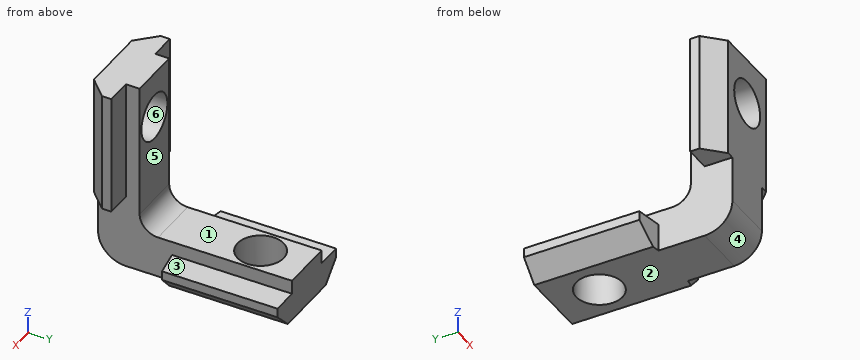
from build123d import *

# Parameters (mm, degrees)
BOSS_EXTRUDE1_DEPTH      = 13
SKETCH2_R                = 2.5
CUT_EXTRUDE1_DEPTH       = 23.207487476
BOSS_EXTRUDE2_DEPTH      = 13
CUT_EXTRUDE2_DEPTH       = 28.297847901
BOSS_EXTRUDE3_DEPTH      = 2.85
BOSS_EXTRUDE3_DEPTH_BACK = 2.85
SKETCH5_W                = 4.5
SKETCH5_H                = 2.5


with BuildPart() as part:
    # Sketch1 → Boss-Extrude1 (new body)
    with BuildSketch(Plane.XY.offset(21)):
        Polygon((-2.85, 4.5), (2.85, 4.5), (2.85, 3), (5.65, 3), (5.65, 2), (3.65, 0), (-3.65, 0), (-5.65, 2), (-5.65, 3), (-2.85, 3), align=None)
    extrude(amount=-BOSS_EXTRUDE1_DEPTH)

    # Sketch2 → Cut-Extrude1 (cut, through all)
    with BuildSketch(Plane(origin=(0, 4.5, 0), x_dir=(1, 0, 0), z_dir=(0, 1, 0))):
        with Locations(Location((0, -16, 0), (0, 0, 180))):
            Circle(SKETCH2_R)
    extrude(amount=-CUT_EXTRUDE1_DEPTH, mode=Mode.SUBTRACT)



with BuildPart() as body_2:
    # Sketch3 → Boss-Extrude2 (new body)
    with BuildSketch(Plane(origin=(0, 21, 0), x_dir=(-1, 0, 0), z_dir=(0, 1, 0))):
        Polygon((2.85, 4.5), (-2.85, 4.5), (-2.85, 3), (-5.65, 3), (-5.65, 2), (-3.65, 0), (3.65, 0), (5.65, 2), (5.65, 3), (2.85, 3), align=None)
    extrude(amount=-BOSS_EXTRUDE2_DEPTH)

    # Sketch6 → Cut-Extrude2 (cut, through all)
    with BuildSketch(Plane.XY.offset(4.5)):
        Polygon((-5.65, 8), (-5.65, 8.5), (-2.85, 8), align=None)
        Polygon((2.85, 8), (5.65, 8), (5.65, 8.5), align=None)
    extrude(amount=-CUT_EXTRUDE2_DEPTH, mode=Mode.SUBTRACT)


with BuildPart() as part_1:
    add(part.part)

    add(body_2.part)  # Boss-Extrude3 merges body 2
    # Sketch7 → Boss-Extrude3 (add, two sides: drawn at the far end of the back side and taken through both)
    with BuildSketch(Plane(origin=(0, 0, 0), x_dir=(0, 0, -1), z_dir=(1, 0, 0)).offset(-BOSS_EXTRUDE3_DEPTH_BACK)):
        with BuildLine():
            Line((-8, 0), (-3, 0))
            ThreePointArc((-3, 0), (-0.878679656, 0.878679656), (0, 3))
            Line((0, 3), (0, 8))
            Line((0, 8), (-4.5, 8))
            Line((-4.5, 8), (-4.5, 6.5))
            ThreePointArc((-4.5, 6.5), (-5.085786438, 5.085786438), (-6.5, 4.5))
            Line((-6.5, 4.5), (-8, 4.5))
            Line((-8, 4.5), (-8, 0))
        make_face()
    extrude(amount=BOSS_EXTRUDE3_DEPTH + BOSS_EXTRUDE3_DEPTH_BACK)

    # Sketch5 → Cut-Revolve1 (revolve, cut)
    with BuildSketch(Plane(origin=(0, 0, 0), x_dir=(0, 0, -1), z_dir=(1, 0, 0)), mode=Mode.PRIVATE) as cut_revolve1_sk:
        with Locations((-2.25, 17.25)):
            Rectangle(SKETCH5_W, SKETCH5_H)
    revolve(cut_revolve1_sk.sketch.rotate(Axis((0, 16, 6.063446942), (0, 0, -1)), 90), axis=Axis((0, 16, 6.063446942), (0, 0, -1)), mode=Mode.SUBTRACT)


solid = part_1.part
Work out the finished part from the listing and answer in its coordinate system (mm). Face numbers are marked on the shaded views. A direction names the side the tool comes from. Give positions to 0.01 mm unless a question says otherwise; leave off trailing zeros. Order: outer loops, then holes, each group sorted by start corner. A loop starts at its lowest first (then second) coordinate and runs counter-clockwise, first axis right, second up. Notation, with made-up numbers: (61.5, -34) -> (76.5, -34) arc R26 ccw to (76.5, -11) -> close; hole circle Ø11 at (58.25, 11.25). An arc over 180 degrees is marked (long way). One line per item, written item: value.
Item 1: A tool of negligible diameter and unlimited length cuts with its end or side. For the marked faces 1, 2 and 3, from which of +Z, -Z, +X, -X, +Y, -Y can it reach the whole face along a straight path? Write none if from no direction.
Answer sheet:
face 1: +Z, +X, -X, +Y
face 2: -Z, +X, -X, +Y, -Y
face 3: +Z, +X, +Y, -Y
Item 2: Flat-ended cylindrical pins translate along their axes: P1, Ø4.5, axis at x = -0.5, z = 13, coming from the +Y side; P2, Ø1, axis at x = 3, y = 12.5, coming from the +Z side; P3, Ø0.8, axis at x = -4.5, z = 12.5, coming from the +Y side. Find the tip coordinate at first contact, or state that the pin passes through.
Answer sheet:
P1: y = 4.5
P2: z = 4.5
P3: y = 3
Item 3: Find section A-A, the plane x = -1.5. Give the vertices of the cut face in (y, z).
Answer sheet:
outline: (0, 3) arc R3 ccw to (3, 0) -> (14, 0) -> (14, 4.5) -> (6.5, 4.5) arc R2 cw to (4.5, 6.5) -> (4.5, 14) -> (0, 14) -> close; (0, 18) -> (4.5, 18) -> (4.5, 21) -> (0, 21) -> close; (18, 0) -> (21, 0) -> (21, 4.5) -> (18, 4.5) -> close
Item 4: Straight lines are drawn through the part: probe 1 along X at (y, z) = (16, 2.55); probe 2 along Y at (x, z) = (3, 11.75); probe 3 along Y at (x, z) = (0, 1.35). For each, find the intervals that lie inside material, in ascending order.
Answer sheet:
probe 1: -5.65 to -2.5, 2.5 to 5.65
probe 2: 0 to 3
probe 3: 0.49 to 13.5, 18.5 to 21
Item 5: Determine the mould class of the marked faces 4, 5 and 6 for opening direction Z: released by +Z, released by -Z, zero draft, split by the parting line, or undercut.
Answer sheet:
face 4: released by -Z
face 5: zero draft
face 6: undercut
Item 6: Find section B-B, the plane y = 16. Give the vertices of the cut face in (x, z).
Answer sheet:
outline: (-5.65, 2) -> (-3.65, 0) -> (-2.5, 0) -> (-2.5, 4.5) -> (-2.85, 4.5) -> (-2.85, 3) -> (-5.65, 3) -> close; (2.5, 0) -> (3.65, 0) -> (5.65, 2) -> (5.65, 3) -> (2.85, 3) -> (2.85, 4.5) -> (2.5, 4.5) -> close
Item 7: Find section D-D, the plane x = -4.5. Give the vertices of the cut face in (y, z).
Answer sheet:
outline: (0.85, 8) -> (3, 8) -> (3, 21) -> (0.85, 21) -> close; (8.29, 0.85) -> (21, 0.85) -> (21, 3) -> (8.29, 3) -> close
